Input: dimensioned drawing with shaded views. Units: mm. Origin: part minimum x, y, z. Give positions to 0.01 mm unless a question says otherwise; leave off trailing zeros. Loops run counter-clockwise (first coordinate to the right, second up) from the corner with the lowest first, then second, coordinate; pieces in that order, holes last. Notation, with made-up numbers: (-7, 66) -> (51, 66) arc R11 cw to (51, 71) -> close; hole circle Ø2 at (75.25, 23). An arc over 180 degrees is marked (long way). Answer in a Markdown table with one row per item. Add a question column.
1) First-contact query: P1, Ø2, axis at x = 727.5, z = 15, coming from the +Y side; P2, Ø5, axis at x = 454, z = 2.5, coming from the +Y side. Flat tips, straight axial feed; report the tip coordinate or a pass-through.
2) Section query D-D (x = 935). Return the cut outline in (y, z).
3) Section query B-B (x = 653). Return the cut outline in (y, z), plus the area to 3 significant figures.
4) Line query: line 1 (X direction, y = 675, z = 16.75); line 2 (X direction, y = 791, z = 1.25) (1 decimal); line 3 (Y direction, x = 409.5, z = 17.75) (1 decimal). Output: solid intervals per line, ascending. Write a range as from..to.
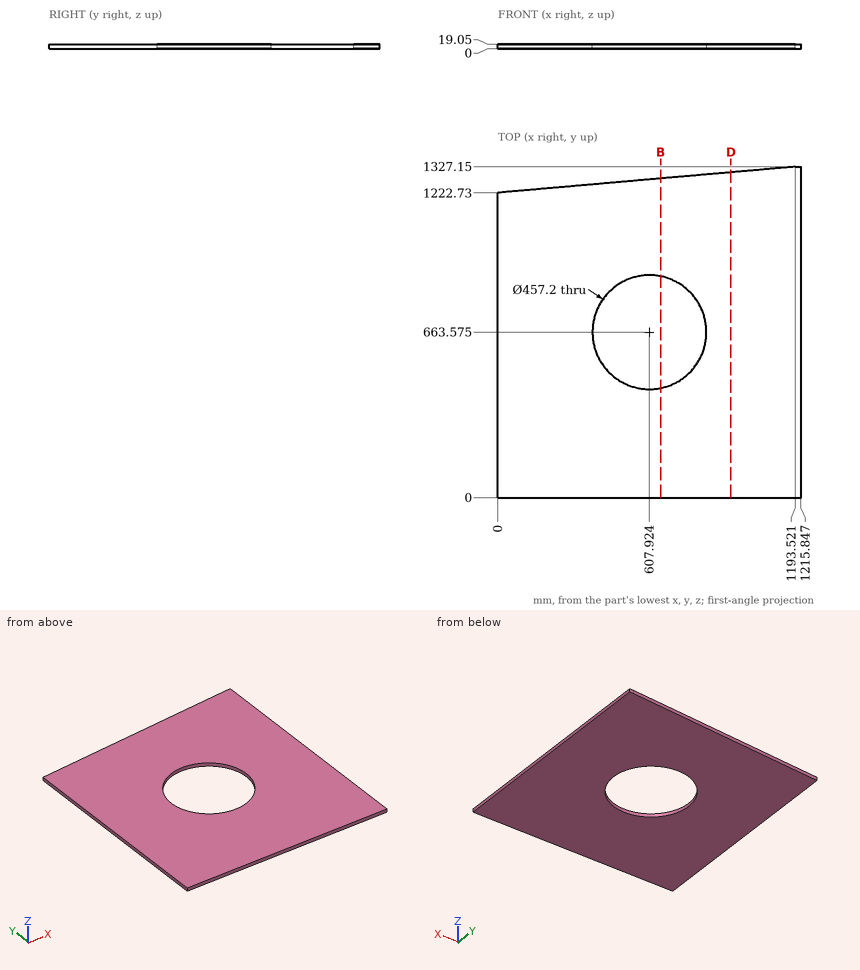
Evaluation:
| question | item | result |
|---|---|---|
| 1 | P1 | y = 1286.47 |
| 1 | P2 | y = 1262.67 |
| 2 | outline | (0, 0) -> (1304.53, 0) -> (1304.53, 19.05) -> (0, 19.05) -> close |
| 3 | outline | (0, 0) -> (439.46, 0) -> (439.46, 19.05) -> (0, 19.05) -> close; (887.69, 0) -> (1279.86, 0) -> (1279.86, 19.05) -> (887.69, 19.05) -> close |
| 3 | area | 15,800 mm² |
| 4 | line 1 | 0..379.61, 836.24..1215.85 |
| 4 | line 2 | 0..418.1, 797.7..1215.8 |
| 4 | line 3 | 0..550.1, 777.1..1258.6 |
